Work out the finished part from the listing and answer in its coordinate system (mm). Give positions to 0.01 mm unless a question says otherwise; leave off trailing zeros. Write each loop counter-clockwise with the first axis right and the second up, starting at its lowest first coordinate (ties: lowest second). Pieces come first, ordered by that corner, then holes. Notation, with made-up numbers: (70.25, -1.5) - (97.25, -1.5) arc R30 cw to (97.25, 23.5) - close; hole circle Ø8 at (-30.75, -24). An arc over 180 degrees is marked (long way). Write item = value, one per line.
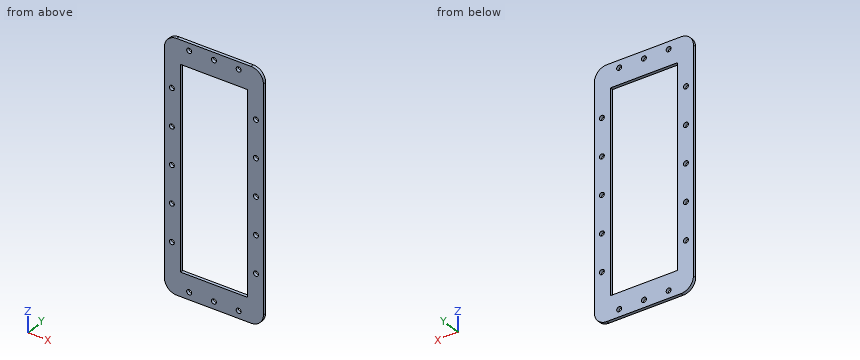
from build123d import *

# Parameters (mm, degrees)
SKETCH1_W           = 101.6
SKETCH1_H           = 254
BOSS_EXTRUDE1_DEPTH = 3.175
SKETCH2_R           = 2.54
CUT_EXTRUDE1_DEPTH  = 223.663234681
FILLET1_R           = 12.7
SKETCH4_W           = 68.631417281
SKETCH4_H           = 205.47036429
CUT_EXTRUDE2_DEPTH  = 223.663234681


with BuildPart() as part:
    # Sketch1 → Boss-Extrude1 (new body)
    with BuildSketch(Plane(origin=(0, 0, 0), x_dir=(1, 0, 0), z_dir=(0, 1, 0))):
        with Locations((20.100372359, -84.049692378)):
            Rectangle(SKETCH1_W, SKETCH1_H)
    extrude(amount=BOSS_EXTRUDE1_DEPTH)

    # Sketch2 → Cut-Extrude1 (cut, through all)
    with BuildSketch(Plane(origin=(0, 3.175, 0), x_dir=(1, 0, 0), z_dir=(0, 1, 0))):
        with Locations(Location((-5.299627641, 35.330307622, 0), (0, 0, 270))):
            Circle(SKETCH2_R)
        with Locations(Location((20.100372359, 35.330307622, 0), (0, 0, 270))):
            Circle(SKETCH2_R)
        with Locations(Location((45.500372359, 35.330307622, 0), (0, 0, 270))):
            Circle(SKETCH2_R)
        with Locations(Location((-23.079627641, -84.049692378, 0), (0, 0, 270))):
            Circle(SKETCH2_R)
        with Locations(Location((-23.079627641, -45.949692378, 0), (0, 0, 270))):
            Circle(SKETCH2_R)
        with Locations(Location((-23.079627641, -7.849692378, 0), (0, 0, 270))):
            Circle(SKETCH2_R)
        with Locations(Location((63.280372359, -7.849692378, 0), (0, 0, 90))):
            Circle(SKETCH2_R)
        with Locations(Location((63.280372359, -45.949692378, 0), (0, 0, 90))):
            Circle(SKETCH2_R)
        with Locations(Location((63.280372359, -84.049692378, 0), (0, 0, 90))):
            Circle(SKETCH2_R)
        with Locations(Location((63.280372359, -122.149692378, 0), (0, 0, 270))):
            Circle(SKETCH2_R)
        with Locations(Location((63.280372359, -160.249692378, 0), (0, 0, 270))):
            Circle(SKETCH2_R)
        with Locations(Location((-23.079627641, -160.249692378, 0), (0, 0, 90))):
            Circle(SKETCH2_R)
        with Locations(Location((-23.079627641, -122.149692378, 0), (0, 0, 90))):
            Circle(SKETCH2_R)
        with Locations(Location((45.500372359, -203.429692378, 0), (0, 0, 90))):
            Circle(SKETCH2_R)
        with Locations(Location((20.100372359, -203.429692378, 0), (0, 0, 90))):
            Circle(SKETCH2_R)
        with Locations(Location((-5.299627641, -203.429692378, 0), (0, 0, 90))):
            Circle(SKETCH2_R)
    extrude(amount=-CUT_EXTRUDE1_DEPTH, mode=Mode.SUBTRACT)

    # Fillet1
    fillet1_edges = [part.edges().sort_by_distance(p)[0] for p in [
        (-30.699627641, 1.5875, -42.950307622),
        (70.900372359, 1.5875, -42.950307622),
        (70.900372359, 1.5875, 211.049692378),
        (-30.699627641, 1.5875, 211.049692378),
    ]]
    fillet(fillet1_edges, radius=FILLET1_R)

    # Sketch4 → Cut-Extrude2 (cut, through all)
    with BuildSketch(Plane(origin=(0, 3.175, 0), x_dir=(1, 0, 0), z_dir=(0, 1, 0))):
        with Locations((20.100372358, -84.049692378)):
            Rectangle(SKETCH4_W, SKETCH4_H)
    extrude(amount=-CUT_EXTRUDE2_DEPTH, mode=Mode.SUBTRACT)


solid = part.part
1. Find section C-C, the plane y = 1.9. Give the number of separate pieces and of enclosed holes in the cut face, then the cut area to 3 significant figures.
Solution:
separate_pieces = 1
enclosed_holes = 17
area = 11,200 mm^2
2. Find section A-A, the plane z = 74.5. Give the vertices of the cut face in (x, y) (3 decimals).
Solution:
outline = (-30.7, 0) - (-14.215, 0) - (-14.215, 3.175) - (-30.7, 3.175) - close; (54.416, 0) - (70.9, 0) - (70.9, 3.175) - (54.416, 3.175) - close
3. Straight lines are drawn through the part: line 1 (Z direction, x = -5.5, y = 0.15); line 2 (Z direction, x = -11.5, y = 0.6); line 3 (X direction, y = 0.55, z = 118). For each, find the intervals that lie inside material, in ascending order.
Solution:
line_1 = -42.95 to -37.86, -32.8 to -18.69, 186.78 to 200.9, 205.96 to 211.05
line_2 = -42.95 to -18.69, 186.78 to 211.05
line_3 = -30.7 to -14.22, 54.42 to 70.9
4. Given pin 1 (3 mm diameter, centred on x = 63.28, z = 45.95, fed in from -Y); pin 2 (6.5 mm diameter, centred on x = -5.3, z = -35.33, fed in from +Y) (3 decimals), each flat-ended and moving along its own axis, determine where each tip first touches the part or whether it passes through.
Solution:
pin_1 = through
pin_2 = 3.175
5. Find section B-B, the plane x = 28.5. Give the vertices of the cut face in (y, z) (3 decimals).
Solution:
outline = (0, -42.95) - (3.175, -42.95) - (3.175, -18.685) - (0, -18.685) - close; (0, 186.785) - (3.175, 186.785) - (3.175, 211.05) - (0, 211.05) - close
